```python
from build123d import *

# Parameters (mm, degrees)
F1_DEPTH = 20
F2_SIZE  = 10
F4_DEPTH = 10


with BuildPart() as f1:
    # F0 (on Top) → F1 (new body)
    with BuildSketch(Plane.XY):
        Polygon((0, 30), (0, -30), (40, -30), (40, -10), (20, -10), (20, 10), (40, 10), (40, 30), align=None)
    extrude(amount=F1_DEPTH)

    # F2
    f2_edges = [f1.edges().sort_by_distance(p)[0] for p in [
        (40, -30, 10),
        (40, 30, 10),
    ]]
    chamfer(f2_edges, length=F2_SIZE)

    # F3 (on face) → F4 (join)
    with BuildSketch(Plane(origin=(0, 0, 0), x_dir=(0, -1, 0), z_dir=(-1, 0, 0))):
        Polygon((-30, 40), (-30, 20), (30, 20), (30, 30), (10, 30), (10, 40), align=None)
    extrude(amount=-F4_DEPTH)


solid = f1.part
```
Input: part model. Units: mm. Frame: model coordinates. A direction names the side the tool comes from. Round coordinates to 2 decimals unless told otherwise and drop trailing zeros. Loops run counter-clockwise (first coordinate to the right, second up) from the corner with the lowest first, then second, coordinate; pieces in that order, holes last. Notation, with made-up numbers: M 55,30.25 L 87,30.25 A18 cw 87,47.25 Z; hole C -38,18.5 d4. An arc over 180 degrees is marked long. Answer in a Markdown table with one row per item. Add a question column.
1. Contact query for flat-ended pins moving along their axis: pin 1 (4 mm diameter, centred on x = 34.5, z = 14, fed in from +Y); pin 2 (11 mm diameter, centred on x = 7.5, y = -18, fed in from +Z); pin 3 (10 mm diameter, centred on y = 12, z = 30.5, fed in from +X). Output: stop coordinate, or through.
2. Ray query, probe 1 along Y at (x, z) = (25, 18); probe 2 along X at (y, z) = (21, 28); probe 3 along Z at (x, y) = (28, 15). Return the intervals inside material, ascending.
3. Section D-D (x = 8). Output: boundary loops of the cut face in (y, z), and give its area (3 significant figures).
4. Set-up query: faces 1 (the face through (30, -10, 10)), 2 (the face through (10, 7, 30)), 3 (the face through (35, -25, 10)), 4 (the face through (35, 25, 10)), 5 (the face through (5, -10, 35)). Return all of +Z, -Z, +X, -X, +Y, -Y with unobstructed straight access to the full face (end or side cutting, diameter ignored); none if empty.
5. Mould query, pull axis Y, two halves, no side actions, for faces 6 (the face through (30, 10, 10)), 7 (the face through (15, -30, 11)), 8 (the face through (18, 0, 20)). Classes: released by +Y, released by -Y, zero draft, split by the parting line, or undercut.
6. Section C-C (z = 3). Output: boundary loops of the cut face in (x, y), and give its area (3 significant figures).
7. Section B-B (y = 6). Output: boundary loops of the cut face in (x, z).
8. Section A-A (x = 26). Output: boundary loops of the cut face in (y, z), and give its area (3 significant figures).
Values follow:
| question | item | result |
|---|---|---|
| 1 | pin 1 | y = 27.5 |
| 1 | pin 2 | z = 30 |
| 1 | pin 3 | x = 10 |
| 2 | probe 1 | -30 to -10, 10 to 30 |
| 2 | probe 2 | 0 to 10 |
| 2 | probe 3 | 0 to 20 |
| 3 | outline | M -30,0 L 30,0 L 30,40 L -10,40 L -10,30 L -30,30 Z |
| 3 | area | 2,200 mm^2 |
| 4 | face 1 | +Z, -Z, +X |
| 4 | face 2 | +Z, +X, +Y, -Y |
| 4 | face 3 | +Z, -Z, +X, -Y |
| 4 | face 4 | +Z, -Z, +X, +Y |
| 4 | face 5 | +Z, +X, -X, -Y |
| 5 | face 6 | undercut |
| 5 | face 7 | released by -Y |
| 5 | face 8 | zero draft |
| 6 | outline | M 0,-30 L 30,-30 L 40,-20 L 40,-10 L 20,-10 L 20,10 L 40,10 L 40,20 L 30,30 L 0,30 Z |
| 6 | area | 1,900 mm^2 |
| 7 | outline | M 0,0 L 20,0 L 20,20 L 10,20 L 10,40 L 0,40 Z |
| 8 | outline | M -30,0 L -10,0 L -10,20 L -30,20 Z; M 10,0 L 30,0 L 30,20 L 10,20 Z |
| 8 | area | 800 mm^2 |
